```python
from build123d import *

# Parameters (mm, degrees)
SKETCH_1_W          = 27
SKETCH_1_H          = 15
EXTRUDE_1_DEPTH     = 7.5
SKETCH_2_R          = 2.25
EXTRUDE_2_DEPTH     = 10
SKETCH_3_R          = 1.5
EXTRUDE_3_DEPTH     = 5
FILLET_1_R          = 2
SKETCH_4_W          = 11
SKETCH_4_H          = 3
CUT_EXTRUDE_1_DEPTH = 10


with BuildPart() as part:
    # Эскиз1 → Бобышка-Вытянуть1 (new body)
    with BuildSketch(Plane(origin=(0, 0, 0), x_dir=(1, 0, 0), z_dir=(0, 1, 0))):
        with Locations((13.5, 7.5)):
            Rectangle(SKETCH_1_W, SKETCH_1_H)
    extrude(amount=EXTRUDE_1_DEPTH)

    # Эскиз2 → Бобышка-Вытянуть2 (add)
    with BuildSketch(Plane(origin=(27, 0, 0), x_dir=(0, 0, -1), z_dir=(1, 0, 0))):
        with Locations(Location((7.5, 3.75, 0), (0, 0, 180))):
            Circle(SKETCH_2_R)
    extrude(amount=EXTRUDE_2_DEPTH)

    # Эскиз3 → Бобышка-Вытянуть3 (add)
    with BuildSketch(Plane(origin=(37, 0, 0), x_dir=(0, 0, -1), z_dir=(1, 0, 0))):
        with Locations((7.5, 3.75)):
            Circle(SKETCH_3_R)
    extrude(amount=EXTRUDE_3_DEPTH)

    # Скругление1
    fillet_1_edges = [part.edges().sort_by_distance(p)[0] for p in [
        (13.5, 7.5, -15),
        (13.5, 7.5, 0),
        (13.5, 0, -15),
        (13.5, 0, 0),
    ]]
    fillet(fillet_1_edges, radius=FILLET_1_R)

    # Эскиз4 → Вырез-Вытянуть1 (cut)
    with BuildSketch(Plane.ZY):
        with Locations((-7.5, 5)):
            Rectangle(SKETCH_4_W, SKETCH_4_H)
    extrude(amount=-CUT_EXTRUDE_1_DEPTH, mode=Mode.SUBTRACT)


solid = part.part
```
CAD build for the part. Positions are in the model's coordinates, mm. A direction names the side the tool comes from. Round coordinates to 2 decimals unless told otherwise and drop trailing zeros. Order: outer loops, then holes, each group sorted by start corner. A loop starts at its lowest first (then second) coordinate and runs counter-clockwise, first axis right, second up.
Item 1: Saw through at A-A on x = 7. Write the cut outline in (y, z).
Item 2: Saw through at B-B on z = -7.5. Write the cut outline in (x, y).
Item 3: Saw through at D-D on y = 3. Write the cut outline in (x, z).
Item 4: Saw through at C-C on x = 17. Write the cut outline in (y, z), then the cut area to 3 significant figures.
Item 5: Pin check, flat tips, straight feed: pin 1 (3 mm diameter, centred on x = 36, y = 4.5, fed in from -Z); pin 2 (0.9 mm diameter, centred on y = 5.5, z = -9, fed in from -X). Stop position of each tip, or through.
Item 6: Probe line 1 along X through (y, z) = (3.25, -4); line 2 along Z through (x, y) = (5.5, 4.75); line 3 along X through (y, z) = (5.25, -11). List the from-to ranges inside material, lowest first.
Item 7: Tool access for faces 1 (the face through (13, 4, -15)), 2 (the face through (5, 5, -13)), 3 (the face through (37, 3, -6)): list every direction of +Z, -Z, +X, -X, +Y, -Y with a clear straight run to the whole face (end or side of a thin tool).
Item 8: Mould opens along Z. For faces 4 (the face through (31.9, 5.1, -9.3)), 5 (the face through (10, 5, -8)), 6 (the face through (13.69, 0.6, -14.43)), 7 (the face through (5, 5, -2)) say: pulls with the +Z half, pulls with the -Z half, needs draft (parallel to the pull), parting line crosses it, or undercut.
Reported:
1. outline: (0, -13) arc R2 ccw to (2, -15) - (5.5, -15) arc R2 ccw to (7.5, -13) - (7.5, -2) arc R2 ccw to (5.5, 0) - (2, 0) arc R2 ccw to (0, -2) - close; hole (3.5, -13) - (6.5, -13) - (6.5, -2) - (3.5, -2) - close
2. outline: (0, 0) - (27, 0) - (27, 1.5) - (37, 1.5) - (37, 2.25) - (42, 2.25) - (42, 5.25) - (37, 5.25) - (37, 6) - (27, 6) - (27, 7.5) - (0, 7.5) - (0, 6.5) - (10, 6.5) - (10, 3.5) - (0, 3.5) - close
3. outline: (0, -15) - (27, -15) - (27, -9.62) - (37, -9.62) - (37, -8.8) - (42, -8.8) - (42, -6.2) - (37, -6.2) - (37, -5.38) - (27, -5.38) - (27, 0) - (0, 0) - close
4. outline: (0, -13) arc R2 ccw to (2, -15) - (5.5, -15) arc R2 ccw to (7.5, -13) - (7.5, -2) arc R2 ccw to (5.5, 0) - (2, 0) arc R2 ccw to (0, -2) - close
4. area: 109 mm2
5. pin 1: stops at z = -9.75
5. pin 2: stops at x = 10
6. line 1: x = 0 to 27
6. line 2: z = -15 to -13, -2 to 0
6. line 3: x = 10 to 27
7. face 1: -Z, +X, -X, +Y, -Y
7. face 2: -X
7. face 3: +X
8. face 4: parting line crosses it
8. face 5: undercut
8. face 6: pulls with the -Z half
8. face 7: undercut
